Build history of the part. All positions in model axes, mm. A direction names the side the tool comes from. Round coordinates to 2 decimals unless told otherwise and drop trailing zeros. Write each loop counter-clockwise with the first axis right and the second up, starting at its lowest first coordinate (ties: lowest second). Pieces come first, ordered by that corner, then holes. Notation, with made-up numbers: (45.5, 41.5) -> (89.5, 41.5) arc R30 ccw to (89.5, 78.5) -> close; hole circle Ø11 at (-6, 38). An arc over 180 degrees is marked (long way). Answer as CSV lines item,"result".
from build123d import *

# Parameters (mm, degrees)
F2_SIZE  = 0.6
F3_R     = 2
F4_DEPTH = 26
F5_R     = 1.5
F6_DEPTH = 10


with BuildPart() as f1:
    # F0 (on Top) → F1 (revolve)
    with BuildSketch(Plane.XY):
        with BuildLine():
            Line((0, 21.5), (0, 0))
            Line((0, 0), (16, 0))
            Line((16, 0), (16, 7.5))
            Line((16, 7.5), (4, 7.5))
            ThreePointArc((4, 7.5), (2.918364, 10.189654), (4, 12.879307))
            Line((4, 12.879307), (4, 21.5))
            Line((4, 21.5), (0, 21.5))
        make_face()
        with BuildLine():
            Line((16, 0), (0, 0))
            Line((0, 0), (0, -21.5))
            Line((0, -21.5), (4, -21.5))
            Line((4, -21.5), (4, -12.879307))
            ThreePointArc((4, -12.879307), (2.918364, -10.189654), (4, -7.5))
            Line((4, -7.5), (16, -7.5))
            Line((16, -7.5), (16, 0))
        make_face()
    revolve(axis=Axis((0, 10.75, 0), (0, -1, 0)))

    # F2
    f2_edges = [f1.edges().sort_by_distance(p)[0] for p in [
        (-4, 21.5, 0),
        (-16, 7.5, 0),
        (-16, -7.5, 0),
        (-4, -21.5, 0),
    ]]
    chamfer(f2_edges, length=F2_SIZE)

    # F3 (on Top) → F4 (join)
    with BuildSketch(Plane.XY):
        Circle(F3_R)
    extrude(amount=F4_DEPTH)

    # F5 (on face) → F6 (cut)
    with BuildSketch(Plane.XY.offset(26)):
        Circle(F5_R)
    extrude(amount=-F6_DEPTH, mode=Mode.SUBTRACT)


solid = f1.part
1. Drop flat-ended pins along their axis: pin 1 Ø8 at (x, z) = (11, -10.5) entering from -Y; pin 2 Ø8 at (y, z) = (16, 9) entering from +X; pin 3 Ø8 at (y, z) = (7.5, -10.5) entering from -X; pin 4 Ø1.5 at (y, z) = (3, 10.5) entering from +X. Give the stop position or say it passes through.
Results found:
pin 1,"stops at y = -7.5"
pin 2,"passes through"
pin 3,"stops at x = -14.6"
pin 4,"stops at x = 12.69"
2. Mould opens along X. For faces 5 (the flat face through (0, 0, 16)), 6 (the cylindrical face through (-0.867, 16.946, -3.905)), 7 (the flat face through (0, 21.5, 0)) say: +X half, -X half, draft (parallel to the pull), parting line (faces both ways), or undercut.
Results found:
face 5,"undercut"
face 6,"parting line"
face 7,"draft"
3. Probe line 1 along Y through (x, z) = (0, 18); line 2 along X through (y, z) = (3.5, -0.5); line 3 along Y through (x, z) = (12.5, 7). List the from-to ranges inside material, lowest first.
Results found:
line 1,"y = -2 to -1.5, 1.5 to 2"
line 2,"x = -15.99 to 15.99"
line 3,"y = -7.5 to 7.5"
4. Cut at D-D, the plane z = 17.5. Write the cut outline in (x, y).
Results found:
outline,"circle Ø4 at (0, 0); hole circle Ø3 at (0, 0)"
5. Which spindle directions (+Z, -Z, +X, -X, +Y, -Y) get a long thin tool onto all of the face, cutting with end or side? Do faces 1 (the flat face through (0, -21.5, 0)), 2 (the cylindrical face through (0, -2, 21)), 3 (the flat face through (3, 7.5, -3)), 4 (the flat face through (-3, -7.5, -3)). Say none if no direction does.
Results found:
face 1,"+Z, -Z, +X, -X, -Y"
face 2,"+Z"
face 3,"+Y"
face 4,"-Y"
6. Cut at C-C, the plane y = 0. Write the cut outline in (x, z).
Results found:
outline,"(-2, 15.87) arc R16 ccw (long way) to (2, 15.87) -> (2, 26) -> (1.5, 26) -> (1.5, 16) -> (-1.5, 16) -> (-1.5, 26) -> (-2, 26) -> close"
7. Cut at B-B, the plane z = 0. Write the cut outline in (x, y).
Results found:
outline,"(-16, -6.9) -> (-15.4, -7.5) -> (-4, -7.5) arc R3.88 cw to (-4, -12.88) -> (-4, -20.9) -> (-3.4, -21.5) -> (3.4, -21.5) -> (4, -20.9) -> (4, -12.88) arc R3.88 cw to (4, -7.5) -> (15.4, -7.5) -> (16, -6.9) -> (16, 6.9) -> (15.4, 7.5) -> (4, 7.5) arc R3.88 cw to (4, 12.88) -> (4, 20.9) -> (3.4, 21.5) -> (-3.4, 21.5) -> (-4, 20.9) -> (-4, 12.88) arc R3.88 cw to (-4, 7.5) -> (-15.4, 7.5) -> (-16, 6.9) -> close"
